For this review, take the finished solid that the model builds, in its own axes (mm). Round coordinates to 2 decimals unless told otherwise and drop trailing zeros. Loops run counter-clockwise (first coordinate to the right, second up) from the corner with the lowest first, then second, coordinate; pieces in that order, holes last. Notation, with made-up numbers: (-23, -33) -> (-16, -33) arc R26 ccw to (-16, -9) -> close; hole circle Ø5 at (-6, -11.5). An arc over 180 degrees is marked (long way). One line per question, with ' | ' between items. Start each with the question number.
1. Consider section A-A (y = -1.75). Write out the cut boundary in (x, z), and give its area (3 significant figures).
2. For pin 1 Ø3 at (y, z) = (-3, 81) entering from +X; pin 2 Ø3 at (y, z) = (-2, 75) entering from -X; pin 3 Ø2 at (y, z) = (-5.5, 47) entering from +X, all flat-tipped, find the tip position at first contact; note any pin that passes through.
3. Consider section C-C (z = 52). Write out the cut boundary in (x, y).
4. Wall thickness on line 1 along Z through (x, y) = (82, -4.75); line 2 along X through (y, z) = (-5.5, 9.5); line 3 along X through (y, z) = (-3.25, 46.5): over which ranges is each line inside the solid? List them lowest first.
5. Consider section B-B (x = 84.5). Write out the cut boundary in (y, z).
```python
from build123d import *

# Parameters (mm, degrees)
F1_DEPTH = 6.35


with BuildPart() as f1:
    # F0 (on Front) → F1 (new body)
    with BuildSketch(Plane.XZ):
        with BuildLine():
            Line((21.332435, 18.212982), (21.332435, 0))
            Line((21.332435, 0), (56.653813, 0))
            ThreePointArc((56.653813, 0), (59.137729, 0.505972), (61.225805, 1.943257))
            Line((61.225805, 1.943257), (68.496529, 9.486627))
            ThreePointArc((68.496529, 9.486627), (70.584605, 10.923911), (73.068521, 11.429884))
            Line((73.068521, 11.429884), (111.03247, 11.429884))
            ThreePointArc((111.03247, 11.429884), (115.522598, 13.289755), (117.38247, 17.779884))
            Line((117.38247, 17.779884), (117.38247, 27.849807))
            ThreePointArc((117.38247, 27.849807), (116.677864, 32.982936), (114.616169, 37.736345))
            Line((114.616169, 37.736345), (103.733808, 55.660222))
            ThreePointArc((103.733808, 55.660222), (101.950588, 59.506153), (101.062049, 63.651216))
            Line((101.062049, 63.651216), (97.911447, 95.157258))
            Line((97.911447, 95.157258), (36.912486, 95.157258))
            Line((36.912486, 95.157258), (36.912486, 66.70589))
            Line((36.912486, 66.70589), (24.837947, 43.530565))
            Line((24.837947, 43.530565), (21.332435, 18.212982))
        make_face()
    extrude(amount=F1_DEPTH)


solid = f1.part
```
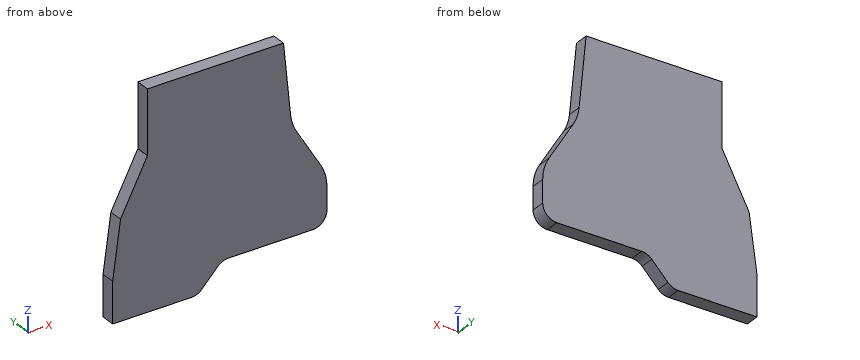
Answer block:
1) outline: (21.33, 0) -> (56.65, 0) arc R6.35 ccw to (61.23, 1.94) -> (68.5, 9.49) arc R6.35 cw to (73.07, 11.43) -> (111.03, 11.43) arc R6.35 ccw to (117.38, 17.78) -> (117.38, 27.85) arc R19.05 ccw to (114.62, 37.74) -> (103.73, 55.66) arc R19.05 cw to (101.06, 63.65) -> (97.91, 95.16) -> (36.91, 95.16) -> (36.91, 66.71) -> (24.84, 43.53) -> (21.33, 18.21) -> close | area: 6,980 mm2
2) pin 1: stops at x = 99.48 | pin 2: stops at x = 36.91 | pin 3: stops at x = 109.6
3) outline: (29.25, -6.35) -> (105.96, -6.35) -> (105.96, 0) -> (29.25, 0) -> close
4) line 1: z = 11.43 to 95.16 | line 2: x = 21.33 to 68.51 | line 3: x = 26.39 to 109.3
5) outline: (-6.35, 11.43) -> (0, 11.43) -> (0, 95.16) -> (-6.35, 95.16) -> close
